Part print with two shaded views. Sizes in mm from the minimum x, y, z corner. Round coordinates to 2 decimals unless told otherwise and drop trailing zeros. Write each loop counter-clockwise with the first axis right and the second up, starting at its lowest first coordinate (ties: lowest second). Pieces come first, ordered by that corner, then holes. Notation, with made-up numbers: (-40, 42) -> (7, 42) arc R17 ccw to (7, 58) -> close; hole circle Ø9 at (65.5, -28.75). An arc over 180 degrees is marked (long way). Put each result on its own line as item: value. Start each with the question number.
1. Saw through at A-A on y = 71. List the corners of the cut face in (x, z) (1 decimal), and give its area (3 significant figures).
2. Saw through at B-B on x = 2.25. State how many separate pieces and enclosed holes the cut face has, and give its area (3 significant figures).
3. Drill centre lines: line 1 (Z direction, x = 0.8, y = 14.5); line 2 (Y direction, x = 0.35, z = 91.5); line 3 (Y direction, x = 2.25, z = 77) (1 decimal). Where is each one in solid material? Low to high. Write a range as from..to.
4. Flat gauge pin, fed straight in: P1, Ø1, axis at x = 1.5, z = 42.5, coming from the +Y side. Where does the tip first touch, or does it go through?
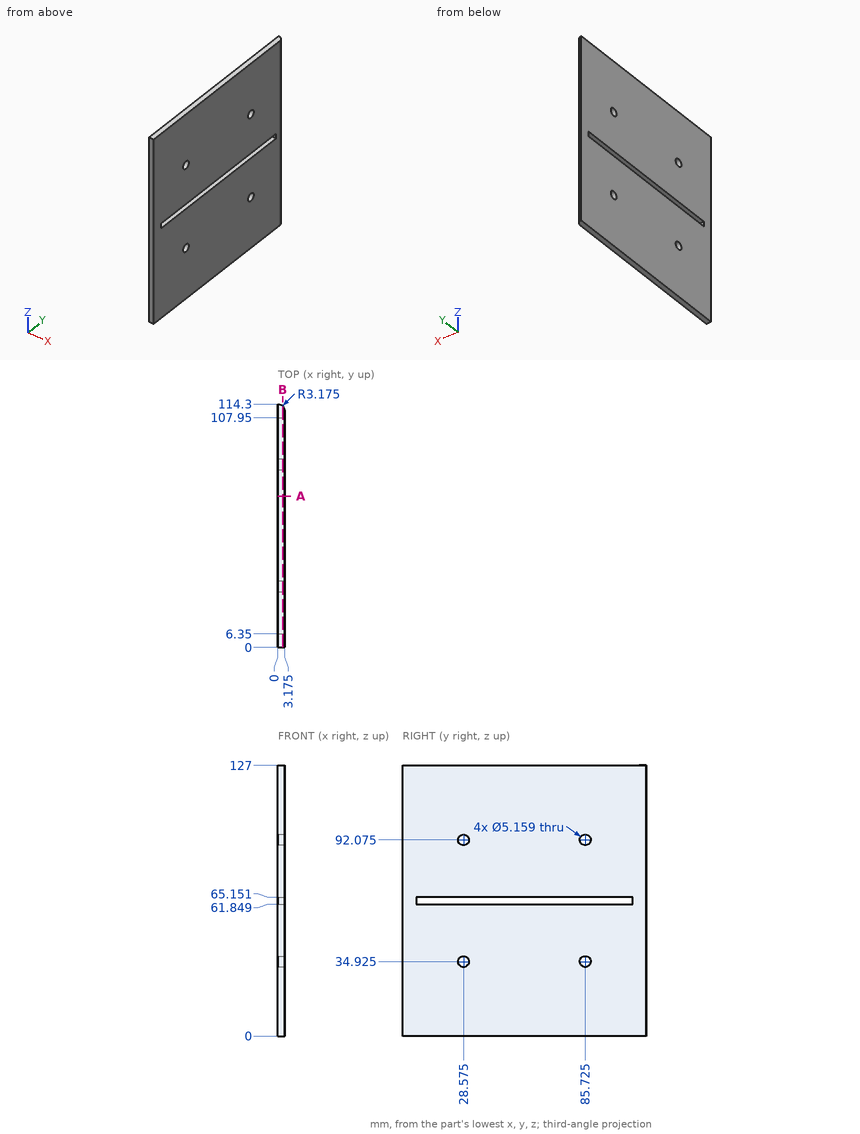
Return value:
1. outline: (0, 0) -> (3.2, 0) -> (3.2, 61.8) -> (0, 61.8) -> close; (0, 65.2) -> (3.2, 65.2) -> (3.2, 127) -> (0, 127) -> close
1. area: 393 mm^2
2. separate pieces: 1
2. enclosed holes: 5
2. area: 14,000 mm^2
3. line 1: z = 0..61.85, 65.15..127
3. line 2: y = 0..26.06, 31.09..83.21, 88.24..114.28
3. line 3: y = 0..113.4
4. P1: stops at y = 114.14
